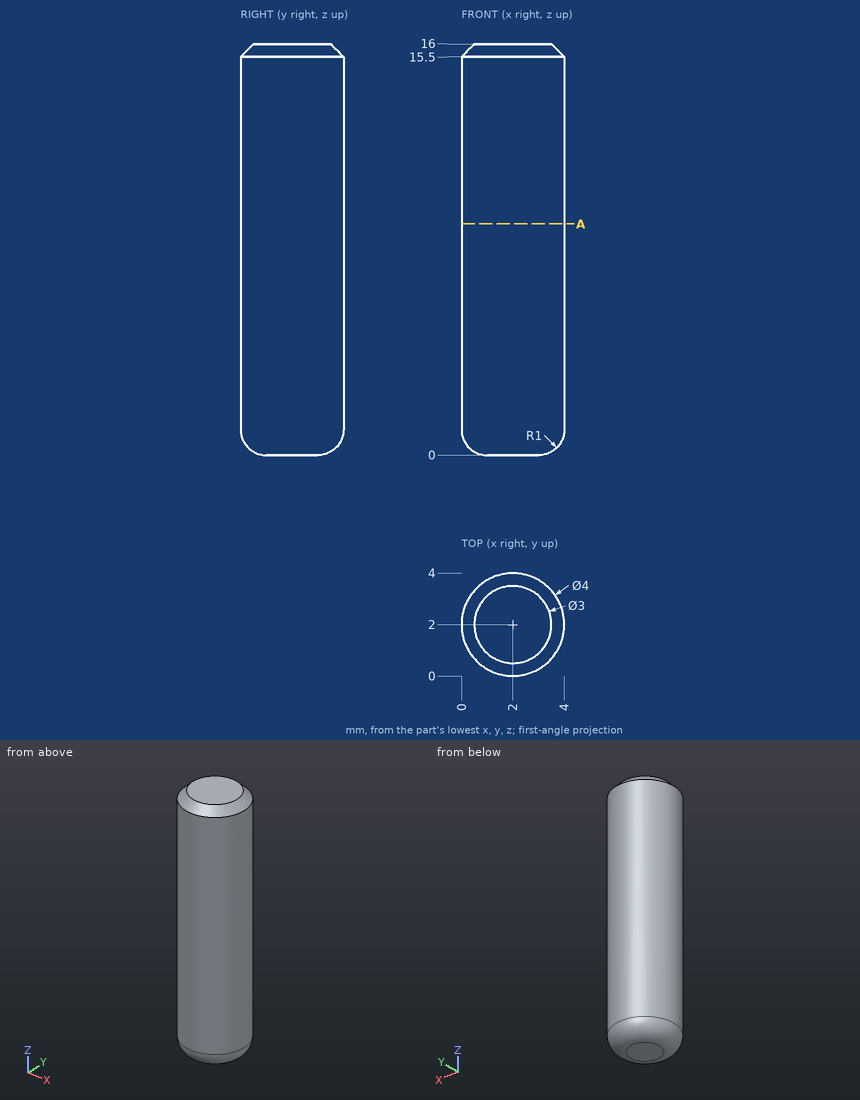
Input: dimensioned drawing with shaded views. Units: mm. Origin: part minimum x, y, z. Round coordinates to 2 decimals unless told otherwise and drop trailing zeros. Loops run counter-clockwise (first coordinate to the right, second up) from the corner with the lowest first, then second, coordinate; pieces in that order, holes last. Notation, with made-up numbers: M 75,42.25 L 100,42.25 A18 cw 100,75.25 Z; hole C 74.5,69.25 d10. An arc over 180 degrees is marked long. Return JSON: item names as keys, results as strings. Group by question number.
1. Section query A-A on z = 9. Output: boundary loops of the cut face in (x, y).
2. Pin query (flat end, axial travel): pin 1 (1.5 mm diameter, centred on x = 1.5, z = 6, fed in from +Y); pin 2 (1.5 mm diameter, centred on y = 0.5, z = 10.5, fed in from +X). Return the tip coordinate at first contact, or that it passes through.
3. Material intervals for line 1 along Z through (x, y) = (2.55, 1); line 2 along X through (y, z) = (2.75, 3.5); line 3 along Z through (x, y) = (3.05, 3.2), sorted ascending. Write a range as from..to.
Checks:
{
 "1": {"outline": "C 2,2 d4"},
 "2": {"pin 1": "stops at y = 4", "pin 2": "stops at x = 3.85"},
 "3": {"line 1": "z = 0.01..16", "line 2": "x = 0.15..3.85", "line 3": "z = 0.2..15.91"}
}
